Can you work these out from the model? Positions are in its coordinate system, mm. A direction names the side the tool comes from. Round coordinates to 2 decimals unless told otherwise and drop trailing zeros. Loops run counter-clockwise (first coordinate to the right, second up) from the corner with the lowest first, then second, coordinate; pieces in that order, holes last. Notation, with made-up numbers: (-24, -31.75) - (10, -31.75) arc R31 cw to (10, 3.25) - close; hole circle Ø4 at (23.5, -3). An arc over 180 degrees is marked (long way). Answer as CSV lines item,"result".
```python
from build123d import *

# Parameters (mm, degrees)
F0_W     = 150.972114
F0_H     = 82.764328
F1_DEPTH = 1
F3_DEPTH = 25
F4_R     = 5.447895
F4_R_2   = 6.606543
F4_R_3   = 6.639495
F5_DEPTH = 25


with BuildPart() as f1:
    # F0 (on Top) → F1 (new body)
    with BuildSketch(Plane.XY):
        Rectangle(F0_W, F0_H)
    extrude(amount=F1_DEPTH)

    # F2 (on face) → F3 (cut)
    with BuildSketch(Plane.XY.offset(1)):
        Polygon((-75.486057, 14.666528), (75.486057, 41.382164), (-75.486057, 41.382164), align=None)
        Polygon((-52.455958, -13.873742), (-75.486057, 14.666528), (-75.486057, -22.594379), align=None)
        Polygon((-75.486057, -41.382164), (75.486057, -41.382164), (-75.486057, -22.594379), align=None)
    extrude(amount=-F3_DEPTH, mode=Mode.SUBTRACT)

    # F4 (on face) → F5 (cut)
    with BuildSketch(Plane.XY.offset(1)):
        with Locations((32.90059, 13.609481)):
            Circle(F4_R)
        with Locations((29.729448, -14.402266)):
            Circle(F4_R_2)
        with Locations((-22.065856, 0)):
            Circle(F4_R_3)
    extrude(amount=-F5_DEPTH, mode=Mode.SUBTRACT)


solid = f1.part
```
Q1. On a 3-axis mill with a long thin cutter (end or side, diameter ignored), from which of +Z, -Z, +X, -X, +Y, -Y can I reach the whole of each face in a straight line? I mean faces 4 (the cylindrical face through (-15.73, 1.99, 0.51)), 5 (the flat face through (-64.132, -18.295, 0.507)). Say none if no direction works.
Checks:
face 4,"+Z, -Z"
face 5,"+Z, -Z, -X"
Q2. Imagine slicing it at A-A (x = 26). Write out the boundary of the cut face in (y, z).
Checks:
outline,"(-35.22, 0) - (-19.86, 0) - (-19.86, 1) - (-35.22, 1) - close; (-8.95, 0) - (32.63, 0) - (32.63, 1) - (-8.95, 1) - close"
Q3. Imagine slicing it at C-C (y = -5). Write out the boundary of the cut face in (x, z), then the cut area to 3 significant figures.
Checks:
outline,"(-59.62, 0) - (-26.43, 0) - (-26.43, 1) - (-59.62, 1) - close; (-17.7, 0) - (75.49, 0) - (75.49, 1) - (-17.7, 1) - close"
area,"126 mm²"
Q4. I'm going to push a flat-ended pin straight in: pin 1 Ø12 at (x, y) = (-22.07, 0) entering from +Z. Where does the tip first touch, or does it pass through?
Checks:
pin 1,"through"
Q5. Imagine slicing it at D-D (x = -36.5). Write out the boundary of the cut face in (y, z), then the cut area to 3 significant figures.
Checks:
outline,"(-27.45, 0) - (21.57, 0) - (21.57, 1) - (-27.45, 1) - close"
area,"49.0 mm²"
Q6. We'd pull the mould along X, two halves only. Please class faces 1 (the flat face through (-1.057, 27.837, 0.507)), 2 (the cylindrical face through (38.097, 15.246, 0.507)), 3 (the flat face through (16, 1, 0)): pulls with the +X half, pulls with the -X half, needs draft (parallel to the pull), parting line crosses it, or undercut.
Checks:
face 1,"pulls with the -X half"
face 2,"undercut"
face 3,"needs draft"
Q7. If I drill on line 1 along Y through (x, z) = (32.5, 0.35); line 2 along Y through (x, z) = (37, 0.7); line 3 along Y through (x, z) = (-63.5, 0.55), over which ranges is the centre line in solid material (lowest first)? Write a range as [from, to].
Checks:
line 1,"[-36.03, -20.4], [-8.4, 8.18], [19.04, 33.78]"
line 2,"[-36.59, 10.02], [17.2, 34.57]"
line 3,"[-24.09, -18.06], [-0.19, 16.79]"
Q8. Imagine slicing it at B-B (z = 0.75). Write out the boundary of the cut face in (x, y), then the cut area to 3 significant figures.
Checks:
outline,"(-75.49, -22.59) - (75.49, -41.38) - (75.49, 41.38) - (-75.49, 14.67) - (-52.46, -13.87) - close; hole circle Ø13.28 at (-22.07, 0); hole circle Ø13.21 at (29.73, -14.4); hole circle Ø10.9 at (32.9, 13.61)"
area,"8,260 mm²"
